Read the model definition and answer for the solid it produces. Units are mm, in the model's axes. A direction names the side the tool comes from. Round coordinates to 2 decimals unless told otherwise and drop trailing zeros. Order: outer loops, then holes, each group sorted by start corner. A loop starts at its lowest first (then second) coordinate and runs counter-clockwise, first axis right, second up. Notation, with made-up numbers: (29.5, 21.5) -> (80.5, 21.5) arc R13 cw to (80.5, 34.5) -> close; hole circle Ø11 at (77.5, -9.75). An arc over 180 degrees is marked (long way). Use a Markdown table: item, result. Add a question column.
1. Given pin 1 (3.5 mm diameter, centred on y = 102.5, z = 0, fed in from -X); pin 2 (1.5 mm diameter, centred on x = -9, y = 74.5, fed in from -Z); pin 3 (1.5 mm diameter, centred on y = 52, z = -0.5, fed in from +X), each flat-ended and moving along its own axis, determine where each tip first touches the part or whether it passes through.
2. Section B-B, the plane x = 26 is taken. Give the vertices of the cut face in (y, z), then the cut area to 3 significant figures.
3. Section C-C, the plane z = -25 is taken. Give the vertices of the cut face in (x, y), then the cut area to 3 significant figures.
4. Consider L1, parallel to Y at x = 10, z = 35; L2, parallel to Z at x = -2, y = 332.5; L3, parallel to X at y = 422, z = -3. Determine where each line is inside the solid, lowest interval first. Write a range as [from, to].
5. For faces 4 (the face through (-23.122, 351.135, -30.156)), 5 (the face through (-1.5, 76.8, 38.4)), 6 (the face through (-38.4, 76.8, 1.5)), determine the directions among +Z, -Z, +X, -X, +Y, -Y from which every point of the face is accessible in a straight line to the end or side of a thin tool.
6. The mould has two halves that part along Y. Classify faces 1 (the face through (-38.4, 76.8, -1.5)), 2 (the face through (18.3, 0, 9.4)), 3 (the face through (-19.524, 152.465, 4.336)): +Y half, -Y half, draft (parallel to the pull), parting line (faces both ways), or undercut.
7. Section A-A, the plane y = 59.5 is taken. Give the vertices of the cut face in (x, z), then the cut area to 3 significant figures.
8. Section D-D, the plane y = 261.5 is taken. Give the vertices of the cut face in (x, z).
```python
from build123d import *

# Parameters (mm, degrees)
SKETCH1_R           = 40
SKETCH1_R_2         = 38
BOSS_EXTRUDE1_DEPTH = 450
SKETCH3_R           = 38
SKETCH3_R_2         = 20
BOSS_EXTRUDE2_DEPTH = 5
LPATTERN1_COUNT     = 5
LPATTERN1_PITCH     = 50
BOSS_EXTRUDE3_START = -10
SKETCH6_R           = 38
BOSS_EXTRUDE3_DEPTH = 10
SKETCH2_W           = 3
SKETCH2_H           = 105
CUT_EXTRUDE6_DEPTH  = 10
CIRPATTERN6_COUNT   = 4


with BuildPart() as part:
    # Sketch1 → Boss-Extrude1 (new body)
    with BuildSketch(Plane(origin=(0, 0, 0), x_dir=(1, 0, 0), z_dir=(0, 1, 0))):
        with Locations(Location((0, 0, 0), (0, 0, 270))):
            Circle(SKETCH1_R)
        with Locations(Location((0, 0, 0), (0, 0, 270))):
            Circle(SKETCH1_R_2, mode=Mode.SUBTRACT)
    extrude(amount=BOSS_EXTRUDE1_DEPTH)

    # Sketch3 → Boss-Extrude2 (add)
    with BuildSketch(Plane.XZ):
        with Locations(Location((0, 0, 0), (0, 0, 270))):
            Circle(SKETCH3_R)
        with Locations(Location((0, 0, 0), (0, 0, 270))):
            Circle(SKETCH3_R_2, mode=Mode.SUBTRACT)
    boss_extrude2 = extrude(amount=-BOSS_EXTRUDE2_DEPTH)

    # LPattern1: Boss-Extrude2 ×5
    with Locations(*[(0, i * LPATTERN1_PITCH, 0) for i in range(1, LPATTERN1_COUNT)]):
        add(boss_extrude2)

    # Sketch6 → Boss-Extrude3 (add)
    with BuildSketch(Plane(origin=(0, 255, 0), x_dir=(1, 0, 0), z_dir=(0, 1, 0)).offset(BOSS_EXTRUDE3_START)):
        with Locations(Location((0, 0, 0), (0, 0, 90))):
            Circle(SKETCH6_R)
    extrude(amount=BOSS_EXTRUDE3_DEPTH)

    # Sketch2 → Cut-Extrude6 (cut)
    with BuildSketch(Plane.ZY.offset(40)):
        with Locations((0, 77.5)):
            Rectangle(SKETCH2_W, SKETCH2_H)
    cut_extrude6 = extrude(amount=-CUT_EXTRUDE6_DEPTH, mode=Mode.SUBTRACT)

    # CirPattern6: Cut-Extrude6 ×4 about axis
    cirpattern6_axis = Axis((0, 0, 0), (0, 1, 0))
    for i in range(1, CIRPATTERN6_COUNT):
        add(cut_extrude6.rotate(cirpattern6_axis, i * 360 / CIRPATTERN6_COUNT), mode=Mode.SUBTRACT)


solid = part.part
```
Verdict:
| question | item | result |
|---|---|---|
| 1 | pin 1 | stops at x = -39.97 |
| 1 | pin 2 | stops at z = -39.14 |
| 1 | pin 3 | stops at x = 30 |
| 2 | outline | (0, -30.4) -> (450, -30.4) -> (450, -27.71) -> (255, -27.71) -> (255, 27.71) -> (450, 27.71) -> (450, 30.4) -> (0, 30.4) -> close; hole (5, -27.71) -> (50, -27.71) -> (50, 27.71) -> (5, 27.71) -> close; hole (55, -27.71) -> (100, -27.71) -> (100, 27.71) -> (55, 27.71) -> close; hole (105, -27.71) -> (150, -27.71) -> (150, 27.71) -> (105, 27.71) -> close; hole (155, -27.71) -> (200, -27.71) -> (200, 27.71) -> (155, 27.71) -> close; hole (205, -27.71) -> (245, -27.71) -> (245, 27.71) -> (205, 27.71) -> close |
| 2 | area | 4,360 mm2 |
| 3 | outline | (-31.22, 0) -> (31.22, 0) -> (31.22, 450) -> (28.62, 450) -> (28.62, 255) -> (-28.62, 255) -> (-28.62, 450) -> (-31.22, 450) -> close; hole (-28.62, 5) -> (28.62, 5) -> (28.62, 50) -> (-28.62, 50) -> close; hole (-28.62, 55) -> (28.62, 55) -> (28.62, 100) -> (-28.62, 100) -> close; hole (-28.62, 105) -> (28.62, 105) -> (28.62, 150) -> (-28.62, 150) -> close; hole (-28.62, 155) -> (28.62, 155) -> (28.62, 200) -> (-28.62, 200) -> close; hole (-28.62, 205) -> (28.62, 205) -> (28.62, 245) -> (-28.62, 245) -> close |
| 3 | area | 4,350 mm2 |
| 4 | L1 | y = [0, 5], [50, 55], [100, 105], [150, 155], [200, 205], [245, 255] |
| 4 | L2 | z = [-39.95, -37.95], [37.95, 39.95] |
| 4 | L3 | x = [-39.89, -37.88], [37.88, 39.89] |
| 5 | face 4 | +Y |
| 5 | face 5 | +Z |
| 5 | face 6 | -X |
| 6 | face 1 | undercut |
| 6 | face 2 | -Y half |
| 6 | face 3 | draft |
| 7 | outline | (-39.97, -1.5) arc R40 ccw to (-1.5, -39.97) -> (-1.5, -37.97) arc R38 cw to (-37.97, -1.5) -> close; (-39.97, 1.5) -> (-37.97, 1.5) arc R38 cw to (-1.5, 37.97) -> (-1.5, 39.97) arc R40 ccw to start; (1.5, -39.97) arc R40 ccw to (39.97, -1.5) -> (37.97, -1.5) arc R38 cw to (1.5, -37.97) -> close; (1.5, 37.97) arc R38 cw to (37.97, 1.5) -> (39.97, 1.5) arc R40 ccw to (1.5, 39.97) -> close |
| 7 | area | 466 mm2 |
| 8 | outline | circle Ø80 at (0, 0); hole circle Ø76 at (0, 0) |
